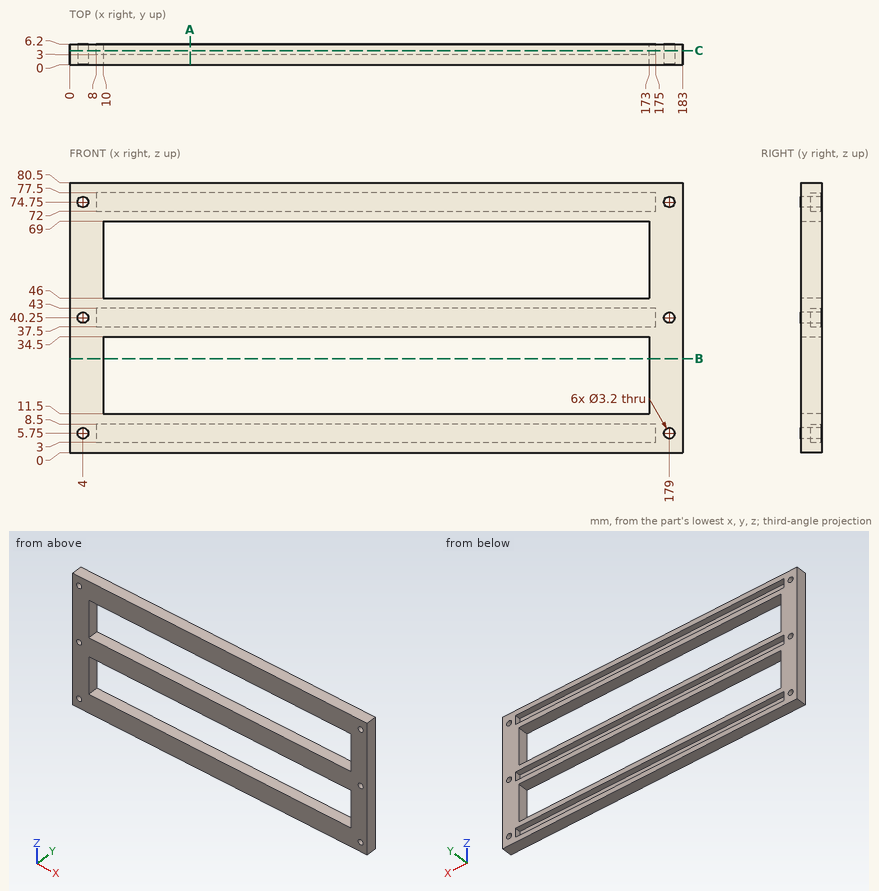
Job drawing, mm, ordinate dimensions from the low corner. One solid piece. Round coordinates to 2 decimals unless told otherwise and drop trailing zeros. Order: outer loops, then holes, each group sorted by start corner. A loop starts at its lowest first (then second) coordinate and runs counter-clockwise, first axis right, second up. Notation, with made-up numbers: (59, 16.5) -> (89, 16.5) arc R15 cw to (89, 37.5) -> close; hole circle Ø10 at (73.5, -8). An arc over 180 degrees is marked (long way). Answer in a Markdown table with one row per item.
1) Band-saw the part on B-B on z = 28. Give the cut face in (x, y), and give its area (3 significant figures).
Values:
| item | result |
|---|---|
| outline | (0, 0) -> (10, 0) -> (10, 6.2) -> (0, 6.2) -> close; (173, 0) -> (183, 0) -> (183, 6.2) -> (173, 6.2) -> close |
| area | 124 mm2 |
2) Band-saw the part on A-A on x = 36. Give the cut face in (y, z).
Values:
| item | result |
|---|---|
| outline | (0, 0) -> (6.2, 0) -> (6.2, 3) -> (3, 3) -> (3, 8.5) -> (6.2, 8.5) -> (6.2, 11.5) -> (0, 11.5) -> close; (0, 34.5) -> (6.2, 34.5) -> (6.2, 37.5) -> (3, 37.5) -> (3, 43) -> (6.2, 43) -> (6.2, 46) -> (0, 46) -> close; (0, 69) -> (6.2, 69) -> (6.2, 72) -> (3, 72) -> (3, 77.5) -> (6.2, 77.5) -> (6.2, 80.5) -> (0, 80.5) -> close |
3) Pin check, flat tips, straight feed: P1, Ø3, axis at y = 3.5, z = 56.5, coming from the -X side; P2, Ø12, axis at x = 65, z = 21.5, coming from the -Y side. Stop position of each tip, or through.
Values:
| item | result |
|---|---|
| P1 | x = 0 |
| P2 | through |
4) Wall check: L1, parallel to Z at x = 137, y = 1; L2, parallel to Z at x = 4, y = 1.75; L3, parallel to Z at x = 75.5, y = 4. Give the ranges that are in metal, low to high.
Values:
| item | result |
|---|---|
| L1 | 0 to 11.5, 34.5 to 46, 69 to 80.5 |
| L2 | 0 to 4.15, 7.35 to 38.65, 41.85 to 73.15, 76.35 to 80.5 |
| L3 | 0 to 3, 8.5 to 11.5, 34.5 to 37.5, 43 to 46, 69 to 72, 77.5 to 80.5 |
5) Band-saw the part on C-C on y = 4.25. Give the number of separate pieces and of enclosed holes in the cut face, and give its area (3 significant figures).
Values:
| item | result |
|---|---|
| separate pieces | 1 |
| enclosed holes | 11 |
| area | 4,430 mm2 |
